Design review of the part built by this model. Coordinates are the model's own, in mm. Face numbers are marked on the shaded views. A direction names the side the tool comes from. Coordinates: 2 decimals unless noted, no trailing zeros. Loops run counter-clockwise (first coordinate to the right, second up) from the corner with the lowest first, then second, coordinate; pieces in that order, holes last. Notation, with made-up numbers: (-2.75, 7.5) -> (42.25, 7.5) arc R19 cw to (42.25, 43.5) -> close; hole circle Ø10 at (70, 63.5). An arc over 180 degrees is marked (long way). Use a Markdown table: item, result. Add a question column.
Q1. Draft analysis for pull direction Y (two halves, no side actions). For the marked faces 1, 2 and 3, state which applies: pulls with the +Y half, pulls with the -Y half, needs draft (parallel to the pull), parting line crosses it, or undercut.
Q2. For the marked faces 4, 5 and 6, list the 3-axis set-ups (+Z, -Z, +X, -X, +Y, -Y) from which the entire face can be reached by the end or side of a thin tool; tool diameter is ignored.
Q3. For probe 1 along X at (y, z) = (-14, 108.5); probe 2 along Y at (x, z) = (0, 65); probe 3 along Y at (x, z) = (4, 23), list the stretches that pass through material, from the lowest coordinate up.
Q4. Clearance check with flat-ended pins moving along their axes: pin 1 Ø12 at (x, z) = (19.5, 54.5) entering from +Y; pin 2 Ø2 at (y, z) = (9, 88.5) entering from -X; pin 3 Ø5 at (y, z) = (20, 102.5) entering from -X. State where each tip first meets the part, or that it passes through.
Q5. Take a section at A-A on z = 98.5. Write out the cut boundary in (x, y), plus the area to 3 significant figures.
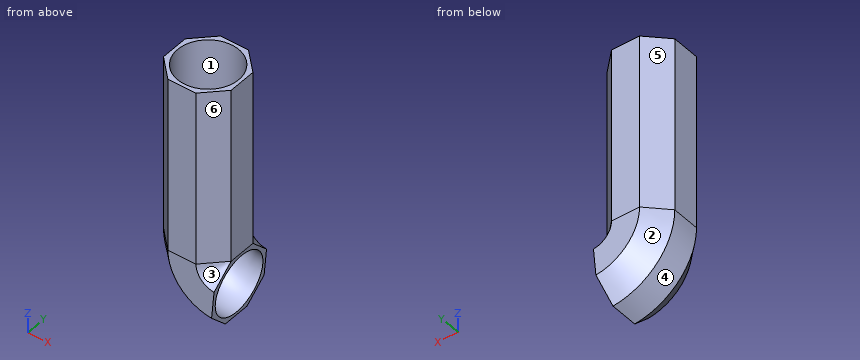
from build123d import *

# Parameters (mm, degrees)
F0_R     = 23.4518638388
F1_ANGLE = 85
F2_DEPTH = 134.62


with BuildPart() as f1:
    # F0 (on Top) → F1 (revolve)
    with BuildSketch(Plane.XY):
        Polygon((25.8333600402, 11.0059764155), (10.4845435083, 26.0493446223), (-11.0059764155, 25.8333600402), (-26.0493446223, 10.4845435083), (-25.8333600402, -11.0059764155), (-10.4845435083, -26.0493446223), (11.0059764155, -25.8333600402), (26.0493446223, -10.4845435083), align=None)
        Circle(F0_R, mode=Mode.SUBTRACT)
    revolve(axis=Axis((25.9413523312, 0.2607164536, 0), (0.0100497185, -0.9999495003, 0)), revolution_arc=F1_ANGLE)

    # F0 (on Top) → F2 (join)
    with BuildSketch(Plane.XY):
        Polygon((25.8333600402, 11.0059764155), (10.4845435083, 26.0493446223), (-11.0059764155, 25.8333600402), (-26.0493446223, 10.4845435083), (-25.8333600402, -11.0059764155), (-10.4845435083, -26.0493446223), (11.0059764155, -25.8333600402), (26.0493446223, -10.4845435083), align=None)
        Circle(F0_R, mode=Mode.SUBTRACT)
    extrude(amount=F2_DEPTH)


solid = f1.part
Answer list:
| question | item | result |
|---|---|---|
| 1 | face 1 | undercut |
| 1 | face 2 | pulls with the +Y half |
| 1 | face 3 | pulls with the -Y half |
| 2 | face 4 | -Z, -X, -Y |
| 2 | face 5 | +Z, -Z, -X, +Y |
| 2 | face 6 | +Z, +X, -Y |
| 3 | probe 1 | -22.78 to -18.81, 18.81 to 22.6 |
| 3 | probe 2 | -25.94 to -23.45, 23.45 to 25.94 |
| 3 | probe 3 | -25.9 to -23.11, 23.11 to 25.98 |
| 4 | pin 1 | y = 23.09 |
| 4 | pin 2 | x = -26.04 |
| 4 | pin 3 | x = -19.17 |
| 5 | outline | (-26.05, 10.48) -> (-25.83, -11.01) -> (-10.48, -26.05) -> (11.01, -25.83) -> (26.05, -10.48) -> (25.83, 11.01) -> (10.48, 26.05) -> (-11.01, 25.83) -> close; hole circle Ø46.9 at (0, 0) |
| 5 | area | 502 mm² |
